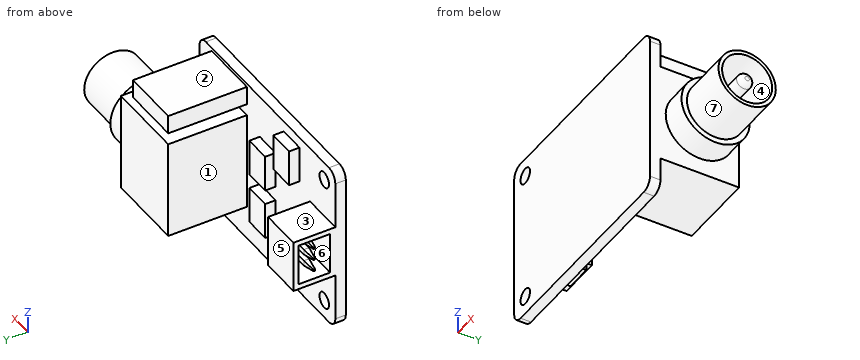
```python
from build123d import *
from OCP.BRepFilletAPI import BRepFilletAPI_MakeChamfer

# Parameters (mm, degrees)
SKETCH1_W           = 43
SKETCH1_H           = 32
SKETCH1_R           = 1.5
BOSS_EXTRUDE1_DEPTH = 2
FILLET1_R           = 2
SKETCH2_W           = 15
SKETCH2_H           = 19
SKETCH2_W_2         = 11.140552481
SKETCH2_H_2         = 3.582781673
BOSS_EXTRUDE2_DEPTH = 15
SKETCH3_W           = 8
SKETCH3_H           = 10
BOSS_EXTRUDE3_DEPTH = 8
SKETCH4_W           = 5
SKETCH4_H           = 7
BOSS_EXTRUDE4_DEPTH = 2
SKETCH5_W           = 8
SKETCH5_H           = 6
SKETCH5_W_2         = 1
SKETCH5_H_2         = 1
CUT_EXTRUDE1_DEPTH  = 7
DRAFT1_ANGLE        = 1
CHAMFER1_SIZE       = 2.5
CHAMFER1_SIZE2      = 0.351352087
CHAMFER1_SIZE2_2    = 0.352269778
CHAMFER1_SIZE2_3    = 0.350545667
SKETCH6_R           = 6.5
BOSS_EXTRUDE5_DEPTH = 5
SKETCH7_R           = 5.464716876
BOSS_EXTRUDE6_DEPTH = 10
SKETCH8_R           = 4.778839206
SKETCH8_R_2         = 1.418417939
CUT_EXTRUDE2_DEPTH  = 15
FILLET3_R           = 1


with BuildPart() as part:
    # Sketch1 → Boss-Extrude1 (new body)
    with BuildSketch(Plane(origin=(0, 0, 0), x_dir=(1, 0, 0), z_dir=(0, 1, 0))):
        with Locations((-157.69047619, 62.928571429)):
            Rectangle(SKETCH1_W, SKETCH1_H)
        with Locations(Location((-175.69047619, 75.428571429, 0), (0, 0, 270))):
            Circle(SKETCH1_R, mode=Mode.SUBTRACT)
        with Locations(Location((-175.69047619, 50.428571429, 0), (0, 0, 270))):
            Circle(SKETCH1_R, mode=Mode.SUBTRACT)
    extrude(amount=BOSS_EXTRUDE1_DEPTH)

    # Fillet1
    fillet1_edges = [part.edges().sort_by_distance(p)[0] for p in [
        (-179.19047619, 1, -78.928571429),
        (-136.19047619, 1, -78.928571429),
        (-136.19047619, 1, -46.928571429),
        (-179.19047619, 1, -46.928571429),
    ]]
    fillet(fillet1_edges, radius=FILLET1_R)

    # Sketch2 → Boss-Extrude2 (add)
    with BuildSketch(Plane(origin=(0, 2, 0), x_dir=(1, 0, 0), z_dir=(0, 1, 0))):
        with Locations((-143.69047619, 62.928571429)):
            Rectangle(SKETCH2_W, SKETCH2_H)
        with Locations((-145.62019995, 49.369059298)):
            Rectangle(SKETCH2_W_2, SKETCH2_H_2)
    extrude(amount=BOSS_EXTRUDE2_DEPTH)

    # Sketch3 → Boss-Extrude3 (add)
    with BuildSketch(Plane(origin=(0, 2, 0), x_dir=(1, 0, 0), z_dir=(0, 1, 0))):
        with Locations((-175.19047619, 62.928571429)):
            Rectangle(SKETCH3_W, SKETCH3_H)
    extrude(amount=BOSS_EXTRUDE3_DEPTH)

    # Sketch4 → Boss-Extrude4 (add)
    with BuildSketch(Plane(origin=(0, 2, 0), x_dir=(1, 0, 0), z_dir=(0, 1, 0))):
        with Locations((-157.781788093, 68.484522729)):
            Rectangle(SKETCH4_W, SKETCH4_H)
        with Locations((-157.781788093, 58.672517023)):
            Rectangle(SKETCH4_W, SKETCH4_H)
        with Locations((-165.512552384, 73.341751138)):
            Rectangle(SKETCH4_W, SKETCH4_H)
        with Locations((-165.361321637, 52.495882076)):
            Rectangle(SKETCH4_W, SKETCH4_H)
    extrude(amount=BOSS_EXTRUDE4_DEPTH)

    # Sketch5 → Cut-Extrude1 (cut)
    with BuildSketch(Plane.ZY.offset(179.19047619)):
        with Locations((-62.928571429, 6)):
            Rectangle(SKETCH5_W, SKETCH5_H)
        with Locations((-65.228571429, 6)):
            Rectangle(SKETCH5_W_2, SKETCH5_H_2, mode=Mode.SUBTRACT)
        with Locations((-62.928571429, 6)):
            Rectangle(SKETCH5_W_2, SKETCH5_H_2, mode=Mode.SUBTRACT)
        with Locations((-60.628571429, 6)):
            Rectangle(SKETCH5_W_2, SKETCH5_H_2, mode=Mode.SUBTRACT)
    extrude(amount=-CUT_EXTRUDE1_DEPTH, mode=Mode.SUBTRACT)

    # Draft1
    draft1_faces = [part.faces().sort_by_distance(p)[0] for p in [
        (-179.19047619, 6, -65.228571429),
        (-179.19047619, 6, -60.628571429),
        (-179.19047619, 6, -62.928571429),
    ]]
    draft(draft1_faces, Plane(origin=(-172.19047619, 6.5, -63.428571429), x_dir=(0, 0, 1), z_dir=(0, 1, 0)), DRAFT1_ANGLE)

    # Chamfer1: one chamfer whose edges measure the first distance from different faces: ONE call of the kernel's chamfer builder (chamfer() names one face for all edges)
    chamfer1_edges_1 = [part.edges().sort_by_distance(p)[0] for p in [
        (-179.199203723, 6, -65.728571429),
    ]]
    chamfer1_side_1 = [part.faces().sort_by_distance(p)[0] for p in [
        (-175.694841768, 5.99979246, -65.728571429),
    ]]
    chamfer1_edges_2 = [part.edges().sort_by_distance(p)[0] for p in [
        (-179.19047619, 6.5, -65.228571429),
    ]]
    chamfer1_side_2 = [part.faces().sort_by_distance(p)[0] for p in [
        (-175.69047619, 6.5, -65.228571429),
    ]]
    chamfer1_edges_3 = [part.edges().sort_by_distance(p)[0] for p in [
        (-179.199203723, 6, -64.728571429),
    ]]
    chamfer1_side_3 = [part.faces().sort_by_distance(p)[0] for p in [
        (-175.694841768, 5.99979246, -64.728571429),
    ]]
    chamfer1_edges_4 = [part.edges().sort_by_distance(p)[0] for p in [
        (-179.207931255, 5.5, -65.228571429),
    ]]
    chamfer1_side_4 = [part.faces().sort_by_distance(p)[0] for p in [
        (-175.699203723, 5.5, -65.228571429),
    ]]
    chamfer1_edges_5 = [part.edges().sort_by_distance(p)[0] for p in [
        (-179.199203723, 6, -63.428571429),
    ]]
    chamfer1_side_5 = [part.faces().sort_by_distance(p)[0] for p in [
        (-175.694841768, 5.99979246, -63.428571429),
    ]]
    chamfer1_edges_6 = [part.edges().sort_by_distance(p)[0] for p in [
        (-179.19047619, 6.5, -62.928571429),
    ]]
    chamfer1_side_6 = [part.faces().sort_by_distance(p)[0] for p in [
        (-175.69047619, 6.5, -62.928571429),
    ]]
    chamfer1_edges_7 = [part.edges().sort_by_distance(p)[0] for p in [
        (-179.199203723, 6, -62.428571429),
    ]]
    chamfer1_side_7 = [part.faces().sort_by_distance(p)[0] for p in [
        (-175.694841768, 5.99979246, -62.428571429),
    ]]
    chamfer1_edges_8 = [part.edges().sort_by_distance(p)[0] for p in [
        (-179.207931255, 5.5, -62.928571429),
    ]]
    chamfer1_side_8 = [part.faces().sort_by_distance(p)[0] for p in [
        (-175.699203723, 5.5, -62.928571429),
    ]]
    chamfer1_edges_9 = [part.edges().sort_by_distance(p)[0] for p in [
        (-179.199203723, 6, -61.128571429),
    ]]
    chamfer1_side_9 = [part.faces().sort_by_distance(p)[0] for p in [
        (-175.694841768, 5.99979246, -61.128571429),
    ]]
    chamfer1_edges_10 = [part.edges().sort_by_distance(p)[0] for p in [
        (-179.19047619, 6.5, -60.628571429),
    ]]
    chamfer1_side_10 = [part.faces().sort_by_distance(p)[0] for p in [
        (-175.69047619, 6.5, -60.628571429),
    ]]
    chamfer1_edges_11 = [part.edges().sort_by_distance(p)[0] for p in [
        (-179.199203723, 6, -60.128571429),
    ]]
    chamfer1_side_11 = [part.faces().sort_by_distance(p)[0] for p in [
        (-175.694841768, 5.99979246, -60.128571429),
    ]]
    chamfer1_edges_12 = [part.edges().sort_by_distance(p)[0] for p in [
        (-179.207931255, 5.5, -60.628571429),
    ]]
    chamfer1_side_12 = [part.faces().sort_by_distance(p)[0] for p in [
        (-175.699203723, 5.5, -60.628571429),
    ]]
    chamfer1 = BRepFilletAPI_MakeChamfer(part.part.solid().wrapped)
    for e in chamfer1_edges_1:
        chamfer1.Add(CHAMFER1_SIZE, CHAMFER1_SIZE2, e.wrapped, chamfer1_side_1[0].wrapped)  # the first distance lies on this face
    for e in chamfer1_edges_2:
        chamfer1.Add(CHAMFER1_SIZE, CHAMFER1_SIZE2_2, e.wrapped, chamfer1_side_2[0].wrapped)  # the first distance lies on this face
    for e in chamfer1_edges_3:
        chamfer1.Add(CHAMFER1_SIZE, CHAMFER1_SIZE2, e.wrapped, chamfer1_side_3[0].wrapped)  # the first distance lies on this face
    for e in chamfer1_edges_4:
        chamfer1.Add(CHAMFER1_SIZE, CHAMFER1_SIZE2_3, e.wrapped, chamfer1_side_4[0].wrapped)  # the first distance lies on this face
    for e in chamfer1_edges_5:
        chamfer1.Add(CHAMFER1_SIZE, CHAMFER1_SIZE2, e.wrapped, chamfer1_side_5[0].wrapped)  # the first distance lies on this face
    for e in chamfer1_edges_6:
        chamfer1.Add(CHAMFER1_SIZE, CHAMFER1_SIZE2_2, e.wrapped, chamfer1_side_6[0].wrapped)  # the first distance lies on this face
    for e in chamfer1_edges_7:
        chamfer1.Add(CHAMFER1_SIZE, CHAMFER1_SIZE2, e.wrapped, chamfer1_side_7[0].wrapped)  # the first distance lies on this face
    for e in chamfer1_edges_8:
        chamfer1.Add(CHAMFER1_SIZE, CHAMFER1_SIZE2_3, e.wrapped, chamfer1_side_8[0].wrapped)  # the first distance lies on this face
    for e in chamfer1_edges_9:
        chamfer1.Add(CHAMFER1_SIZE, CHAMFER1_SIZE2, e.wrapped, chamfer1_side_9[0].wrapped)  # the first distance lies on this face
    for e in chamfer1_edges_10:
        chamfer1.Add(CHAMFER1_SIZE, CHAMFER1_SIZE2_2, e.wrapped, chamfer1_side_10[0].wrapped)  # the first distance lies on this face
    for e in chamfer1_edges_11:
        chamfer1.Add(CHAMFER1_SIZE, CHAMFER1_SIZE2, e.wrapped, chamfer1_side_11[0].wrapped)  # the first distance lies on this face
    for e in chamfer1_edges_12:
        chamfer1.Add(CHAMFER1_SIZE, CHAMFER1_SIZE2_3, e.wrapped, chamfer1_side_12[0].wrapped)  # the first distance lies on this face
    add(Compound.cast(chamfer1.Shape()), mode=Mode.REPLACE)

    # Sketch6 → Boss-Extrude5 (add)
    with BuildSketch(Plane(origin=(-136.19047619, 0, 0), x_dir=(0, 0, -1), z_dir=(1, 0, 0))):
        with Locations(Location((62.928571429, 9.5, 0), (0, 0, 180))):
            Circle(SKETCH6_R)
    extrude(amount=BOSS_EXTRUDE5_DEPTH)

    # Sketch7 → Boss-Extrude6 (add)
    with BuildSketch(Plane(origin=(-131.19047619, 0, 0), x_dir=(0, 0, -1), z_dir=(1, 0, 0))):
        with Locations((62.928571429, 9.5)):
            Circle(SKETCH7_R)
    extrude(amount=BOSS_EXTRUDE6_DEPTH)

    # Sketch8 → Cut-Extrude2 (cut)
    with BuildSketch(Plane(origin=(-121.19047619, 0, 0), x_dir=(0, 0, -1), z_dir=(1, 0, 0))):
        with Locations((62.928571429, 9.5)):
            Circle(SKETCH8_R)
        with Locations((62.928571429, 9.5)):
            Circle(SKETCH8_R_2, mode=Mode.SUBTRACT)
    extrude(amount=-CUT_EXTRUDE2_DEPTH, mode=Mode.SUBTRACT)

    # Fillet3
    fillet3_edges = [part.edges().sort_by_distance(p)[0] for p in [
        (-121.19047619, 9.5, -61.51015349),
    ]]
    fillet(fillet3_edges, radius=FILLET3_R)


solid = part.part
```
Input: part model. Units: mm. Frame: model coordinates. Face numbers are marked on the shaded views. A direction names the side the tool comes from. Round coordinates to 2 decimals unless told otherwise and drop trailing zeros. Loops run counter-clockwise (first coordinate to the right, second up) from the corner with the lowest first, then second, coordinate; pieces in that order, holes last.
1) Section query A-A on x = -135. Return the cut outline in (y, z), plus the area to 3 significant figures.
Ans:
outline: circle Ø13 at (9.5, -62.93); circle Ø2.84 at (9.5, -62.93); hole circle Ø9.56 at (9.5, -62.93)
area: 67.3 mm2
2) Section query C-C on x = -143.5. Return the cut outline in (y, z).
Ans:
outline: (0, -78.93) - (2, -78.93) - (2, -72.43) - (17, -72.43) - (17, -53.43) - (2, -53.43) - (2, -51.16) - (17, -51.16) - (17, -47.58) - (2, -47.58) - (2, -46.93) - (0, -46.93) - close
3) Material intervals for line 1 (X direction, y = 2.5, z = -64); line 2 (Z direction, x = -148.5, y = 14.5); line 3 (Y direction, x = -172.5, z = -62.5), sorted ascending.
Ans:
line 1: x = -179.19 to -171.19, -151.19 to -136.19
line 2: z = -72.43 to -53.43, -51.16 to -47.58
line 3: y = 0 to 3, 5.5 to 6.5, 9 to 10
4) Pull-direction query (Z, two-part tool) for the marked faces 5, 6 and 7; classes: released by +Z, released by -Z, zero draft, split by the parting line, or undercut.
Ans:
face 5: zero draft
face 6: undercut
face 7: split by the parting line
5) Section query D-D on y = 13. Return the cut outline in (x, z).
Ans:
outline: (-151.19, -72.43) - (-136.19, -72.43) - (-136.19, -68.41) - (-131.19, -68.41) - (-131.19, -67.13) - (-121.19, -67.13) - (-121.19, -66.18) - (-136.19, -66.18) - (-136.19, -59.67) - (-121.19, -59.67) - (-121.19, -58.73) - (-131.19, -58.73) - (-131.19, -57.45) - (-136.19, -57.45) - (-136.19, -53.43) - (-151.19, -53.43) - close; (-151.19, -51.16) - (-140.05, -51.16) - (-140.05, -47.58) - (-151.19, -47.58) - close
6) Section query B-B on z = -54. Return the cut outline in (x, y).
Ans:
outline: (-179.19, 0) - (-136.19, 0) - (-136.19, 17) - (-151.19, 17) - (-151.19, 2) - (-162.86, 2) - (-162.86, 4) - (-167.86, 4) - (-167.86, 2) - (-179.19, 2) - close
7) Pin query (flat end, axial travel): pin 1 (0.6 mm diameter, centred on y = 3, z = -67.5, fed in from +X); pin 2 (5 mm diameter, centred on y = 9, z = -51, fed in from -X); pin 3 (1.6 mm diameter, centred on x = -166.5, y = 3.5, fed in from -Z). Return the tip coordinate at first contact, or that it passes through.
Ans:
pin 1: stops at x = -136.19
pin 2: stops at x = -151.19
pin 3: stops at z = -76.84
8) Set-up query: the marked faces 1, 2, 3 and 4. Return all of +Z, -Z, +X, -X, +Y, -Y with unobstructed straight access to the full face (end or side cutting, diameter ignored); none if empty.
Ans:
face 1: +Z, -Z, +Y
face 2: +Z, +X, -X, +Y
face 3: +Z, -X, +Y
face 4: +X
